Geometry: final body of the model. Coordinates: model frame, mm. A direction names the side the tool comes from. Round coordinates to 2 decimals unless told otherwise and drop trailing zeros. Loops run counter-clockwise (first coordinate to the right, second up) from the corner with the lowest first, then second, coordinate; pieces in that order, holes last. Notation, with made-up numbers: (54, 65.5) -> (62, 65.5) arc R28 cw to (62, 90.5) -> close; hole circle Ø8 at (-10, -20.75). An arc over 180 degrees is marked (long way). Answer in a Markdown table with one row per item.
```python
from build123d import *

# Parameters (mm, degrees)
F0_R     = 15
F0_R_2   = 30
F1_DEPTH = 2.5


with BuildPart() as f1:
    # F0 (on Front) → F1 (new body)
    with BuildSketch(Plane.XZ):
        with BuildLine():
            Line((-32.561399, 76.149625), (-2.885725, -124.026205))
            ThreePointArc((-2.885725, -124.026205), (36.209669, -148.109627), (53.237161, -105.465454))
            Line((53.237161, -105.465454), (19.352906, -42.184657))
            ThreePointArc((19.352906, -42.184657), (17.053182, -31.086216), (21.154569, -20.520102))
            Line((21.154569, -20.520102), (74.279384, 48.277464))
            ThreePointArc((74.279384, 48.277464), (41.935595, 143.005296), (-32.561399, 76.149625))
        make_face()
        with Locations((26.789949, -119.626845)):
            Circle(F0_R, mode=Mode.SUBTRACT)
        with Locations((26.789949, 84.948346)):
            Circle(F0_R_2, mode=Mode.SUBTRACT)
    extrude(amount=F1_DEPTH)


solid = f1.part
```
Item 1: Mould query, pull axis X, two halves, no side actions, for faces 1 (the cylindrical face through (43.533, -1.232, 142.565)), 2 (the cylindrical face through (24.837, -1.232, -104.754)), 3 (the flat face through (-17.93, -1.23, -22.54)), 4 (the flat face through (13, -2.5, 0)). Classes: released by +X, released by -X, zero draft, split by the parting line, or undercut.
Ans:
| item | result |
|---|---|
| face 1 | split by the parting line |
| face 2 | undercut |
| face 3 | released by -X |
| face 4 | zero draft |
Item 2: Section query C-C, the plane y = -1.15. Output: boundary loops of the cut face in (x, z), and give its area (3 significant figures).
Ans:
| item | result |
|---|---|
| outline | (-32.56, 76.15) -> (-2.89, -124.03) arc R30 ccw (long way) to (53.24, -105.47) -> (19.35, -42.18) arc R20 cw to (21.15, -20.52) -> (74.28, 48.28) arc R60 ccw (long way) to start; hole circle Ø60 at (26.79, 84.95); hole circle Ø30 at (26.79, -119.63) |
| area | 17,200 mm2 |
Item 3: Set-up query: faces 5 (the cylindrical face through (22.885, -1.232, 114.693)), 6 (the flat face through (47.345, -1.232, 13.397)). Return all of +Z, -Z, +X, -X, +Y, -Y with unobstructed straight access to the full face (end or side cutting, diameter ignored); none if empty.
Ans:
| item | result |
|---|---|
| face 5 | +Y, -Y |
| face 6 | +X, +Y, -Y |
Item 4: Section query D-D, the plane z = -100.5. Output: boundary loops of the cut face in (x, y).
Ans:
| item | result |
|---|---|
| outline | (-6.37, -2.5) -> (50.58, -2.5) -> (50.58, 0) -> (-6.37, 0) -> close |
Item 5: Section query B-B, the plane z = 69. Output: boundary loops of the cut face in (x, y).
Ans:
| item | result |
|---|---|
| outline | (-31.5, -2.5) -> (1.38, -2.5) -> (1.38, 0) -> (-31.5, 0) -> close; (52.2, -2.5) -> (84.63, -2.5) -> (84.63, 0) -> (52.2, 0) -> close |
Item 6: Section query A-A, the plane x = 48. Output: boundary loops of the cut face in (y, z).
Ans:
| item | result |
|---|---|
| outline | (-2.5, -140.84) -> (0, -140.84) -> (0, -95.68) -> (-2.5, -95.68) -> close; (-2.5, 14.25) -> (0, 14.25) -> (0, 63.73) -> (-2.5, 63.73) -> close; (-2.5, 106.16) -> (0, 106.16) -> (0, 141.07) -> (-2.5, 141.07) -> close |
Item 7: Ray query, L1, parallel to Z at x = 46, y = -1.9; L2, parallel to Z at x = 53, y = -1; L3, parallel to Z at x = 25.5, y = -0.55. Return the intervals inside material, ascending.
Ans:
| item | result |
|---|---|
| L1 | -142.67 to -91.95, 11.66 to 61.91, 107.99 to 141.79 |
| L2 | -134.22 to -105.02, 20.72 to 70.35, 99.54 to 138.92 |
| L3 | -149.6 to -134.57, -104.68 to -53.66, -14.89 to 54.98, 114.92 to 144.93 |
